from build123d import *

# Parameters (mm, degrees)
EXTRUDE_1_DEPTH      = 100
EXTRUDE_1_DEPTH_BACK = 50
SKETCH_1_R           = 12.5
SKETCH_2_R           = 15
EXTRUDE_2_DEPTH      = 18
SKETCH_3_R           = 12.5
EXTRUDE_3_DEPTH      = 132
EXTRUDE_START        = 18
SKETCH_4_R           = 15
EXTRUDE_4_DEPTH      = 18
SKETCH_5_R           = 12.5
EXTRUDE_5_DEPTH      = 100
SKETCH_6_R           = 19.05
EXTRUDE_6_DEPTH      = 80
SKETCH_7_R           = 12.5
EXTRUDE_7_DEPTH      = 50
SKETCH_9_R           = 8
EXTRUDE_8_DEPTH      = 20


with BuildPart() as part:
    # 草图1 → 凸台-拉伸1 (new, two sides: drawn at the far end of the back side and taken through both)
    with BuildSketch(Plane(origin=(0, 0, 0), x_dir=(0, 0, -1), z_dir=(1, 0, 0)).offset(-EXTRUDE_1_DEPTH_BACK)):
        Circle(SKETCH_1_R)
    extrude(amount=EXTRUDE_1_DEPTH + EXTRUDE_1_DEPTH_BACK)

    # 草图2 → 凸台-拉伸2 (add)
    with BuildSketch(Plane(origin=(100, 0, 0), x_dir=(0, 0, -1), z_dir=(1, 0, 0))):
        Circle(SKETCH_2_R)
    extrude(amount=-EXTRUDE_2_DEPTH)

    # 草图3 → 凸台-拉伸3 (add)
    with BuildSketch(Plane(origin=(100, 0, 0), x_dir=(0, 0, -1), z_dir=(1, 0, 0))):
        Circle(SKETCH_3_R)
    extrude(amount=EXTRUDE_3_DEPTH)

    # 草图4 → 凸台-拉伸4 (add)
    with BuildSketch(Plane(origin=(232, 0, 0), x_dir=(0, 0, -1), z_dir=(1, 0, 0)).offset(EXTRUDE_START)):
        Circle(SKETCH_4_R)
    extrude(amount=-EXTRUDE_4_DEPTH)

    # 草图5 → 凸台-拉伸5 (add)
    with BuildSketch(Plane(origin=(250, 0, 0), x_dir=(0, 0, -1), z_dir=(1, 0, 0))):
        Circle(SKETCH_5_R)
    extrude(amount=EXTRUDE_5_DEPTH)

    # 草图6 → 凸台-拉伸6 (add)
    with BuildSketch(Plane(origin=(350, 0, 0), x_dir=(0, 0, -1), z_dir=(1, 0, 0))):
        Circle(SKETCH_6_R)
    extrude(amount=EXTRUDE_6_DEPTH)

    # 草图7 → 凸台-拉伸7 (add)
    with BuildSketch(Plane(origin=(430, 0, 0), x_dir=(0, 0, -1), z_dir=(1, 0, 0))):
        Circle(SKETCH_7_R)
    extrude(amount=EXTRUDE_7_DEPTH)

    # 草图9 → 凸台-拉伸8 (add)
    with BuildSketch(Plane(origin=(480, 0, 0), x_dir=(0, 0, -1), z_dir=(1, 0, 0))):
        with Locations((0, -0.60565557)):
            Circle(SKETCH_9_R)
    extrude(amount=EXTRUDE_8_DEPTH)


solid = part.part
Input: part model. Units: mm. Frame: model coordinates. A direction names the side the tool comes from. Give positions to 0.01 mm unless a question says otherwise; leave off trailing zeros. Write each loop counter-clockwise with the first axis right and the second up, starting at its lowest first coordinate (ties: lowest second). Pieces come first, ordered by that corner, then holes. Notation, with made-up numbers: M 19,80.5 L 25,80.5 A13 ccw 25,102.5 Z; hole C -5,49.25 d1. An arc over 180 degrees is marked long. Write item = value, one per line. Start each with the question number.
1) Material intervals for line 1 along X through (y, z) = (9, 11); line 2 along X through (y, z) = (9.5, -16); line 3 along Y through (x, z) = (179.5, 0.5), sorted ascending. Write a range as [from, to].
2) Draft query along X for faces 4 (the cylindrical face through (241.126, 0.66, 14.985)), 5 (the flat face through (350, -12.4, -4)), 6 (the flat face through (250, 12.3, 3.4)), 7 (the flat face through (480, 6, -5)). Return one class per face: +X half, -X half, draft (parallel to the pull), parting line (faces both ways), or undercut.
3) First-contact query: pin 1 Ø10 at (x, y) = (178, 8) entering from +Z; pin 2 Ø1.5 at (x, z) = (36, -4) entering from +Y; pin 3 Ø1 at (y, z) = (0, 14.5) entering from +X. Flat tips, straight axial feed; report the tip coordinate or a pass-through.
4) Cut plane B-B on x = 172. Return the cut outline in (y, z), then the cut area to 3 significant figures.
5) Reachability of faces 1 (the cylindrical face through (15.076, 3.755, -11.923)), 2 (the flat face through (232, 12.3, 3.4)), 3 (the cylindrical face through (454.65, 3.755, -11.923)) from +Z, -Z, +X, -X, +Y, -Y: full face, straight path, thin tool, end or side. Return the list, or none.
Solved:
q1.line_1 = [82, 100], [232, 250], [350, 430]
q1.line_2 = [350, 430]
q1.line_3 = [-12.49, 12.49]
q2.face_4 = draft
q2.face_5 = undercut
q2.face_6 = undercut
q2.face_7 = +X half
q3.pin_1 = 12.13
q3.pin_2 = 12.07
q3.pin_3 = 430
q4.outline = C 0,0 d25
q4.area = 491 mm2
q5.face_1 = -X
q5.face_2 = none
q5.face_3 = +X
